```python
from build123d import *

# Parameters (mm, degrees)
F1_DEPTH = 4.064
F2_W     = 84.829882
F2_H     = 29.745544
F3_DEPTH = 4.826
F4_W     = 6.593369
F4_H     = 17.919544
F5_DEPTH = 27.94


with BuildPart() as f1:
    # F0 (on Top) → F1 (new body)
    with BuildSketch(Plane.XY):
        Polygon((42.414941, 15.974458), (0, 15.974458), (-42.414941, 15.974458), (-42.414941, -13.771086), (0, -13.771086), (42.414941, -13.771086), align=None)
        Polygon((-42.414941, -13.771086), (-42.414941, 15.974458), (-42.414941, 31.122651), (-50.217658, 31.122651), (-50.217658, -29.922441), (-42.414941, -30.020962), align=None)
        Polygon((42.414941, 31.122651), (42.414941, 15.974458), (42.414941, -13.771086), (42.414941, -30.020962), (50.217658, -29.922441), (50.217658, 31.122651), align=None)
    extrude(amount=F1_DEPTH)

    # F2 (on face) → F3 (join)
    with BuildSketch(Plane.XY.offset(4.064)):
        with Locations((0, 1.101686)):
            Rectangle(F2_W, F2_H)
    extrude(amount=F3_DEPTH)

    # F4 (on Top) → F5 (cut)
    with BuildSketch(Plane.XY):
        with Locations((46.333633, 0)):
            Rectangle(F4_W, F4_H)
        with Locations((-46.333633, 0)):
            Rectangle(F4_W, F4_H)
    extrude(amount=F5_DEPTH, mode=Mode.SUBTRACT)


solid = f1.part
```
Build history of the part. All positions in model axes, mm. A direction names the side the tool comes from. Coordinates: 2 decimals unless noted, no trailing zeros. Order: outer loops, then holes, each group sorted by start corner. A loop starts at its lowest first (then second) coordinate and runs counter-clockwise, first axis right, second up. Notation, with made-up numbers: (19.5, 65.5) -> (60.5, 65.5) arc R23 cw to (60.5, 98.5) -> close; hole circle Ø1 at (41.25, 2.5). An arc over 180 degrees is marked (long way). Answer in a Markdown table with one row per item. Add a question column.
Q1. Band-saw the part on D-D, the plane x = 11.5. List the corners of the cut face in (y, z), then the cut area to 3 significant figures.
Q2. Mould opens along Y. For faces 5 (the face through (49.63, 0, 2)), 6 (the face through (50.218, 0, 2)), 7 (the face through (-1, 15.974, 4)) say: +Y half, -Y half, draft (parallel to the pull), parting line (faces both ways), or undercut.
Q3. Band-saw the part on C-C, the plane z = 5.5. List the corners of the cut face in (x, y), then the cut area to 3 significant figures.
Q4. Which spindle directions (+Z, -Z, +X, -X, +Y, -Y) get a long thin tool onto all of the face, cutting with end or side? Do faces 1 (the face through (-49.63, 0, 2)), 2 (the face through (42.415, -22, 2)), 3 (the face through (42.415, 1, 6)), 4 (the face through (42.415, 24, 2)). Say none if no direction does.
Q5. Drop flat-ended pins along their axis: pin 1 (2.5 mm diameter, centred on x = 4, z = 4.5, fed in from -Y); pin 2 (4 mm diameter, centred on y = -10, z = 8, fed in from -X); pin 3 (5 mm diameter, centred on x = 12, z = 1, fed in from +Y). Give the stop position or say it passes through.
Q6. Wall check: line 1 along X through (y, z) = (-2.5, 1.5); line 2 along X through (y, z) = (26, 1.75); line 3 along X through (y, z) = (-9.5, 7). Give the ranges that are in metal, low to high. Write a range as [from, to].
Q7. Band-saw the part on A-A, the plane y = -17. List the corners of the cut face in (x, z), then the cut area to 3 significant figures.
Q8. Band-saw the part on B-B, the plane y = 6.5. List the corners of the cut face in (x, z), then the cut area to 3 significant figures.
Answers follow:
| question | item | result |
|---|---|---|
| 1 | outline | (-13.77, 0) -> (15.97, 0) -> (15.97, 8.89) -> (-13.77, 8.89) -> close |
| 1 | area | 264 mm^2 |
| 2 | face 5 | undercut |
| 2 | face 6 | draft |
| 2 | face 7 | +Y half |
| 3 | outline | (-42.41, -13.77) -> (42.41, -13.77) -> (42.41, 15.97) -> (-42.41, 15.97) -> close |
| 3 | area | 2,520 mm^2 |
| 4 | face 1 | +Z, -Z |
| 4 | face 2 | +Z, -Z, -Y |
| 4 | face 3 | +Z, +X, +Y, -Y |
| 4 | face 4 | +Z, -Z, +Y |
| 5 | pin 1 | y = -13.77 |
| 5 | pin 2 | x = -42.41 |
| 5 | pin 3 | y = 15.97 |
| 6 | line 1 | [-50.22, -49.63], [-43.04, 43.04], [49.63, 50.22] |
| 6 | line 2 | [-50.22, -42.41], [42.41, 50.22] |
| 6 | line 3 | [-42.41, 42.41] |
| 7 | outline | (-50.22, 0) -> (-42.41, 0) -> (-42.41, 4.06) -> (-50.22, 4.06) -> close; (42.41, 0) -> (50.22, 0) -> (50.22, 4.06) -> (42.41, 4.06) -> close |
| 7 | area | 63.4 mm^2 |
| 8 | outline | (-50.22, 0) -> (-49.63, 0) -> (-49.63, 4.06) -> (-50.22, 4.06) -> close; (-43.04, 0) -> (43.04, 0) -> (43.04, 4.06) -> (42.41, 4.06) -> (42.41, 8.89) -> (-42.41, 8.89) -> (-42.41, 4.06) -> (-43.04, 4.06) -> close; (49.63, 0) -> (50.22, 0) -> (50.22, 4.06) -> (49.63, 4.06) -> close |
| 8 | area | 764 mm^2 |
